from build123d import *

# Parameters (mm, degrees)
BOSS_EXTRUDE1_DEPTH      = 415.925
BOSS_EXTRUDE1_DEPTH_BACK = 415.925
CUT_EXTRUDE2_DEPTH       = 48.625
CUT_EXTRUDE2_DEPTH_BACK  = 4.175


with BuildPart() as part:
    # Sketch4 → Boss-Extrude1 (new body, two sides)
    with BuildSketch(Plane.XY) as boss_extrude1_sk:
        with BuildLine():
            Line((-22.225, -18.838333333), (-22.225, 25.4))
            Line((-22.225, 25.4), (-25.4, 25.4))
            Line((-25.4, 25.4), (-25.4, -25.4))
            Line((-25.4, -25.4), (25.4, -25.4))
            Line((25.4, -25.4), (25.4, -22.225))
            Line((25.4, -22.225), (-18.838333333, -22.225))
            ThreePointArc((-18.838333333, -22.225), (-21.233068299, -21.233068299), (-22.225, -18.838333333))
        make_face()
    extrude(amount=BOSS_EXTRUDE1_DEPTH)
    extrude(boss_extrude1_sk.sketch, amount=-BOSS_EXTRUDE1_DEPTH_BACK)

    # Sketch5 → Cut-Extrude2 (cut, two sides)
    with BuildSketch(Plane(origin=(0, -22.225, 0), x_dir=(1, 0, 0), z_dir=(0, 1, 0))) as cut_extrude2_sk:
        Polygon((-25.4, 415.925), (25.4, 365.125), (25.4, 415.925), align=None)
        Polygon((25.4, -415.925), (25.4, -365.125), (-25.4, -415.925), align=None)
    extrude(amount=CUT_EXTRUDE2_DEPTH, mode=Mode.SUBTRACT)
    extrude(cut_extrude2_sk.sketch, amount=-CUT_EXTRUDE2_DEPTH_BACK, mode=Mode.SUBTRACT)


solid = part.part
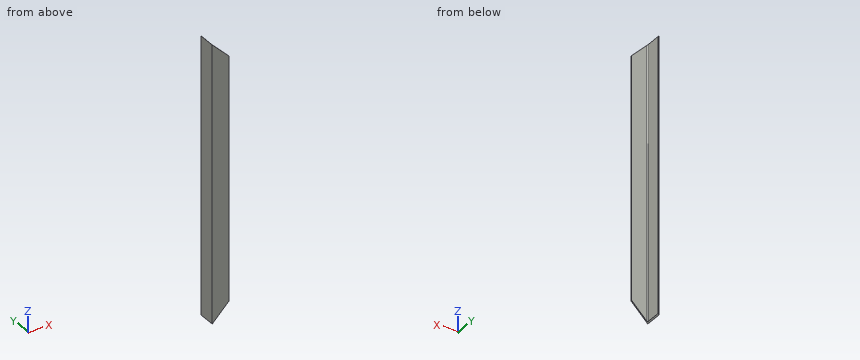
The model under review builds one solid part; all positions refer to its coordinate system, in mm. Coordinates: 2 decimals unless noted, no trailing zeros. Write each loop counter-clockwise with the first axis right and the second up, starting at its lowest first coordinate (ties: lowest second). Pieces come first, ordered by that corner, then holes. Notation, with made-up numbers: (-1.75, 11) - (6.25, 11) arc R16 cw to (6.25, 24) - close; hole circle Ø4 at (45, -4). An arc over 180 degrees is marked (long way). Answer as CSV lines item,"result".
(1) We need section B-B (y = 14.5). Give the boundary of the cut face in (x, z) (3 decimals).
Data:
outline,"(-25.4, -415.925) - (-22.225, -412.75) - (-22.225, 412.75) - (-25.4, 415.925) - close"
(2) For line 1 along Y through (x, z) = (18.5, -252) (3 decimals), list the stretches that pass through material, from the lowest coordinate up. Write a range as [from, to].
Data:
line 1,"y = [-25.4, -22.225]"
(3) We need section C-C (x = -3.5). Give the boundary of the cut face in (y, z) (3 decimals).
Data:
outline,"(-25.4, -394.025) - (-22.225, -394.025) - (-22.225, 394.025) - (-25.4, 394.025) - close"
(4) We need section A-A (z = 114.5). Give the boundary of the cut face in (x, y) (3 decimals), plus the area to 3 significant figures.
Data:
outline,"(-25.4, -25.4) - (25.4, -25.4) - (25.4, -22.225) - (-18.838, -22.225) arc R3.387 cw to (-22.225, -18.838) - (-22.225, 25.4) - (-25.4, 25.4) - close"
area,"315 mm2"
(5) Clearance check with flat-ended pins moving along their axes: pin 1 Ø22 at (y, z) = (-4.5, -179.5) entering from +X (3 decimals); pin 2 Ø13.5 at (x, z) = (4.5, 3) entering from +Y (3 decimals). State where each tip first meets the part, or that it passes through.
Data:
pin 1,"stops at x = -22.225"
pin 2,"stops at y = -22.225"
